from build123d import *

# Parameters (mm, degrees)
SKETCH_1_W      = 15
SKETCH_1_H      = 15
SKETCH_1_R      = 1.25
EXTRUDE_1_DEPTH = 1


with BuildPart() as part:
    # 草图1 → 凸台-拉伸1 (new body)
    with BuildSketch(Plane(origin=(0, 0, 0), x_dir=(1, 0, 0), z_dir=(0, 1, 0))):
        Rectangle(SKETCH_1_W, SKETCH_1_H)
        with Locations((0, -5.5)):
            Circle(SKETCH_1_R, mode=Mode.SUBTRACT)
    extrude(amount=EXTRUDE_1_DEPTH)


solid = part.part
For this review, take the finished solid that the model builds, in its own axes (mm). Round coordinates to 2 decimals unless told otherwise and drop trailing zeros. Order: outer loops, then holes, each group sorted by start corner. A loop starts at its lowest first (then second) coordinate and runs counter-clockwise, first axis right, second up. Notation, with made-up numbers: (32, -1.5) -> (65, -1.5) arc R12 cw to (65, 13.5) -> close; hole circle Ø6 at (78.25, 56.25). An arc over 180 degrees is marked (long way). Put each result on its own line as item: value.
Q1. Insertion check: pin 1 Ø2 at (x, z) = (0, 5.5) entering from +Y. The pin has a flat end and moves straight along its axis. Give the tip position at first contact, or say it passes through.
Check result:
pin 1: through
Q2. For probe 1 along X at (y, z) = (0.6, 5.5); probe 2 along Z at (x, y) = (0, 0.65); probe 3 along X at (y, z) = (0.45, 4.5), list the stretches that pass through material, from the lowest coordinate up. Write a range as [from, to].
Check result:
probe 1: [-7.5, -1.25], [1.25, 7.5]
probe 2: [-7.5, 4.25], [6.75, 7.5]
probe 3: [-7.5, -0.75], [0.75, 7.5]
Q3. Add section A-A on x = 0. Write out the cut boundary in (y, z), plus the area to 3 significant figures.
Check result:
outline: (0, -7.5) -> (1, -7.5) -> (1, 4.25) -> (0, 4.25) -> close; (0, 6.75) -> (1, 6.75) -> (1, 7.5) -> (0, 7.5) -> close
area: 12.5 mm2
Q4. Add section B-B on z = 5.25. Write out the cut boundary in (x, y), plus the area to 3 significant figures.
Check result:
outline: (-7.5, 0) -> (-1.22, 0) -> (-1.22, 1) -> (-7.5, 1) -> close; (1.22, 0) -> (7.5, 0) -> (7.5, 1) -> (1.22, 1) -> close
area: 12.6 mm2
Q5. Mouldability with a two-part tool opening along Z and no side actions: class faces 1 (the flat face through (-0.1, 0.5, -7.5)), 2 (the cylindrical face through (-0.27, 0.49, 6.72)), 3 (the flat face through (7.5, 0.5, 0.1)) as pulls with the +Z half, pulls with the -Z half, needs draft (parallel to the pull), parting line crosses it, or undercut.
Check result:
face 1: pulls with the -Z half
face 2: undercut
face 3: needs draft
